Design review of the part built by this model. Coordinates are the model's own, in mm. A direction names the side the tool comes from. Coordinates: 2 decimals unless noted, no trailing zeros. Write each loop counter-clockwise with the first axis right and the second up, starting at its lowest first coordinate (ties: lowest second). Pieces come first, ordered by that corner, then holes. Notation, with made-up numbers: (19, 44.25) - (67, 44.25) arc R29 ccw to (67, 83.25) - close; hole circle Ø8 at (35, -9). An arc over 180 degrees is marked (long way). Answer as CSV lines item,"result". Start each with the question number.
Q1. Clearance check with flat-ended pins moving along their axes: pin 1 (2.5 mm diameter, centred on x = 0, y = 0, fed in from +Z); pin 2 (3 mm diameter, centred on x = 11.5, z = 4.5, fed in from -Y); pin 3 (1.5 mm diameter, centred on y = -3, z = 2, fed in from +X); pin 4 (3 mm diameter, centred on x = 6.5, z = 5, fed in from +Y). State where each tip first meets the part, or that it passes through.
Q2. We need section A-A (x = 0). Write out the cut boundary in (y, z), plus the area to 3 significant figures.
Q3. For line 1 along Y through (x, z) = (0, 3); line 2 along Y through (x, z) = (-9.5, 3.35); line 3 along X through (y, z) = (13.5, 0.7), list the stretches that pass through material, from the lowest coordinate up. Write a range as [from, to].
Q4. Mouldability with a two-part tool opening along X and no side actions: class faces 4 (the face through (0, 16.5, 3)), 5 (the face through (-5.089, 15.696, 2.712)), 6 (the face through (13.34, -9.71, 2.71)), 7 (the face through (-7.8, -12.8, 2.7)) as pulls with the +X half, pulls with the -X half, needs draft (parallel to the pull), parting line crosses it, or undercut.
Q5. Machinability: for faces 1 (the face through (1.2, -15, 2.7)), 2 (the face through (13.332, -2.12, 2.712)), 3 (the face through (-5.773, -13.85, 2.712)), which of the approach directions +Z, -Z, +X, -X, +Y, -Y give a long, thin tool a straight path to every point of the face, cutting with its end or side? Answer none if there is none.
Q6. We need section D-D (x = 9.5). Write out the cut boundary in (y, z).
Q7. We need section C-C (z = 2.25). State how many separate pieces and enclosed holes the cut face has, plus the area to 3 significant figures.
from build123d import *

# Parameters (mm, degrees)
SKETCH_1_R          = 13.5
EXTRUDE_1_DEPTH     = 5.5
EXTRUDE_START       = -5.5
EXTRUDE_2_DEPTH     = 5.5
SKETCH_7_R          = 2
CUT_EXTRUDE_1_DEPTH = 24.973944189
SKETCH_8_R          = 12.5
SKETCH_8_R_2        = 3
CUT_EXTRUDE_2_DEPTH = 4


with BuildPart() as part:
    # 草图1 → 凸台-拉伸1 (new body)
    with BuildSketch(Plane.XY):
        Circle(SKETCH_1_R)
    extrude(amount=EXTRUDE_1_DEPTH)

    # 草图6 → 凸台-拉伸2 (add)
    with BuildSketch(Plane.XY.offset(5.5).offset(EXTRUDE_START)):
        with BuildLine():
            Line((5.812072794, 15.460669773), (4.38548802, 15.924195265))
            ThreePointArc((4.38548802, 15.924195265), (3.48195608, 14.617198294), (2.719313259, 13.223287617))
            ThreePointArc((2.719313259, 13.223287617), (4.171729424, 12.83926297), (5.572482808, 12.296236634))
            ThreePointArc((5.572482808, 12.296236634), (5.774811944, 13.872204263), (5.812072794, 15.460669773))
        make_face()
        with BuildLine():
            Line((10.305219409, 12.907941468), (9.091693917, 13.789619346))
            ThreePointArc((9.091693917, 13.789619346), (7.828499702, 12.825798085), (6.67244119, 11.735779845))
            ThreePointArc((6.67244119, 11.735779845), (7.935100906, 10.921729424), (9.099492173, 9.972424088))
            ThreePointArc((9.099492173, 9.972424088), (9.778919397, 11.40873523), (10.305219409, 12.907941468))
        make_face()
        with BuildLine():
            Line((0.75, 16.5), (-0.75, 16.5))
            ThreePointArc((-0.75, 16.5), (-1.205425663, 14.97776529), (-1.5, 13.416407865))
            ThreePointArc((-1.5, 13.416407865), (0, 13.5), (1.5, 13.416407865))
            ThreePointArc((1.5, 13.416407865), (1.205425663, 14.97776529), (0.75, 16.5))
        make_face()
        with BuildLine():
            Line((13.789619346, 9.091693917), (12.907941468, 10.305219409))
            ThreePointArc((12.907941468, 10.305219409), (11.40873523, 9.778919397), (9.972424088, 9.099492173))
            ThreePointArc((9.972424088, 9.099492173), (10.921729424, 7.935100906), (11.735779845, 6.67244119))
            ThreePointArc((11.735779845, 6.67244119), (12.825798085, 7.828499702), (13.789619346, 9.091693917))
        make_face()
        with BuildLine():
            Line((15.924195265, 4.38548802), (15.460669773, 5.812072794))
            ThreePointArc((15.460669773, 5.812072794), (13.872204263, 5.774811944), (12.296236634, 5.572482808))
            ThreePointArc((12.296236634, 5.572482808), (12.83926297, 4.171729424), (13.223287617, 2.719313259))
            ThreePointArc((13.223287617, 2.719313259), (14.617198294, 3.48195608), (15.924195265, 4.38548802))
        make_face()
        with BuildLine():
            Line((16.5, -0.75), (16.5, 0.75))
            ThreePointArc((16.5, 0.75), (14.97776529, 1.205425663), (13.416407865, 1.5))
            ThreePointArc((13.416407865, 1.5), (13.5, 0), (13.416407865, -1.5))
            ThreePointArc((13.416407865, -1.5), (14.97776529, -1.205425663), (16.5, -0.75))
        make_face()
        with BuildLine():
            Line((15.460669773, -5.812072794), (15.924195265, -4.38548802))
            ThreePointArc((15.924195265, -4.38548802), (14.617198294, -3.48195608), (13.223287617, -2.719313259))
            ThreePointArc((13.223287617, -2.719313259), (12.83926297, -4.171729424), (12.296236634, -5.572482808))
            ThreePointArc((12.296236634, -5.572482808), (13.872204263, -5.774811944), (15.460669773, -5.812072794))
        make_face()
        with BuildLine():
            Line((12.907941468, -10.305219409), (13.789619346, -9.091693917))
            ThreePointArc((13.789619346, -9.091693917), (12.825798085, -7.828499702), (11.735779845, -6.67244119))
            ThreePointArc((11.735779845, -6.67244119), (10.921729424, -7.935100906), (9.972424088, -9.099492173))
            ThreePointArc((9.972424088, -9.099492173), (11.40873523, -9.778919397), (12.907941468, -10.305219409))
        make_face()
        with BuildLine():
            Line((9.091693917, -13.789619346), (10.305219409, -12.907941468))
            ThreePointArc((10.305219409, -12.907941468), (9.778919397, -11.40873523), (9.099492173, -9.972424088))
            ThreePointArc((9.099492173, -9.972424088), (7.935100906, -10.921729424), (6.67244119, -11.735779845))
            ThreePointArc((6.67244119, -11.735779845), (7.828499702, -12.825798085), (9.091693917, -13.789619346))
        make_face()
        with BuildLine():
            Line((4.38548802, -15.924195265), (5.812072794, -15.460669773))
            ThreePointArc((5.812072794, -15.460669773), (5.774811944, -13.872204263), (5.572482808, -12.296236634))
            ThreePointArc((5.572482808, -12.296236634), (4.171729424, -12.83926297), (2.719313259, -13.223287617))
            ThreePointArc((2.719313259, -13.223287617), (3.48195608, -14.617198294), (4.38548802, -15.924195265))
        make_face()
        with BuildLine():
            Line((-0.75, -16.5), (0.75, -16.5))
            ThreePointArc((0.75, -16.5), (1.205425663, -14.97776529), (1.5, -13.416407865))
            ThreePointArc((1.5, -13.416407865), (0, -13.5), (-1.5, -13.416407865))
            ThreePointArc((-1.5, -13.416407865), (-1.205425663, -14.97776529), (-0.75, -16.5))
        make_face()
        with BuildLine():
            Line((-5.812072794, -15.460669773), (-4.38548802, -15.924195265))
            ThreePointArc((-4.38548802, -15.924195265), (-3.48195608, -14.617198294), (-2.719313259, -13.223287617))
            ThreePointArc((-2.719313259, -13.223287617), (-4.171729424, -12.83926297), (-5.572482808, -12.296236634))
            ThreePointArc((-5.572482808, -12.296236634), (-5.774811944, -13.872204263), (-5.812072794, -15.460669773))
        make_face()
        with BuildLine():
            Line((-10.305219409, -12.907941468), (-9.091693917, -13.789619346))
            ThreePointArc((-9.091693917, -13.789619346), (-7.828499702, -12.825798085), (-6.67244119, -11.735779845))
            ThreePointArc((-6.67244119, -11.735779845), (-7.935100906, -10.921729424), (-9.099492173, -9.972424088))
            ThreePointArc((-9.099492173, -9.972424088), (-9.778919397, -11.40873523), (-10.305219409, -12.907941468))
        make_face()
        with BuildLine():
            Line((-13.789619346, -9.091693917), (-12.907941468, -10.305219409))
            ThreePointArc((-12.907941468, -10.305219409), (-11.40873523, -9.778919397), (-9.972424088, -9.099492173))
            ThreePointArc((-9.972424088, -9.099492173), (-10.921729424, -7.935100906), (-11.735779845, -6.67244119))
            ThreePointArc((-11.735779845, -6.67244119), (-12.825798085, -7.828499702), (-13.789619346, -9.091693917))
        make_face()
        with BuildLine():
            Line((-15.924195265, -4.38548802), (-15.460669773, -5.812072794))
            ThreePointArc((-15.460669773, -5.812072794), (-13.872204263, -5.774811944), (-12.296236634, -5.572482808))
            ThreePointArc((-12.296236634, -5.572482808), (-12.83926297, -4.171729424), (-13.223287617, -2.719313259))
            ThreePointArc((-13.223287617, -2.719313259), (-14.617198294, -3.48195608), (-15.924195265, -4.38548802))
        make_face()
        with BuildLine():
            Line((-16.5, 0.75), (-16.5, -0.75))
            ThreePointArc((-16.5, -0.75), (-14.97776529, -1.205425663), (-13.416407865, -1.5))
            ThreePointArc((-13.416407865, -1.5), (-13.5, 0), (-13.416407865, 1.5))
            ThreePointArc((-13.416407865, 1.5), (-14.97776529, 1.205425663), (-16.5, 0.75))
        make_face()
        with BuildLine():
            Line((-15.460669773, 5.812072794), (-15.924195265, 4.38548802))
            ThreePointArc((-15.924195265, 4.38548802), (-14.617198294, 3.48195608), (-13.223287617, 2.719313259))
            ThreePointArc((-13.223287617, 2.719313259), (-12.83926297, 4.171729424), (-12.296236634, 5.572482808))
            ThreePointArc((-12.296236634, 5.572482808), (-13.872204263, 5.774811944), (-15.460669773, 5.812072794))
        make_face()
        with BuildLine():
            Line((-12.907941468, 10.305219409), (-13.789619346, 9.091693917))
            ThreePointArc((-13.789619346, 9.091693917), (-12.825798085, 7.828499702), (-11.735779845, 6.67244119))
            ThreePointArc((-11.735779845, 6.67244119), (-10.921729424, 7.935100906), (-9.972424088, 9.099492173))
            ThreePointArc((-9.972424088, 9.099492173), (-11.40873523, 9.778919397), (-12.907941468, 10.305219409))
        make_face()
        with BuildLine():
            Line((-9.091693917, 13.789619346), (-10.305219409, 12.907941468))
            ThreePointArc((-10.305219409, 12.907941468), (-9.778919397, 11.40873523), (-9.099492173, 9.972424088))
            ThreePointArc((-9.099492173, 9.972424088), (-7.935100906, 10.921729424), (-6.67244119, 11.735779845))
            ThreePointArc((-6.67244119, 11.735779845), (-7.828499702, 12.825798085), (-9.091693917, 13.789619346))
        make_face()
        with BuildLine():
            Line((-4.38548802, 15.924195265), (-5.812072794, 15.460669773))
            ThreePointArc((-5.812072794, 15.460669773), (-5.774811944, 13.872204263), (-5.572482808, 12.296236634))
            ThreePointArc((-5.572482808, 12.296236634), (-4.171729424, 12.83926297), (-2.719313259, 13.223287617))
            ThreePointArc((-2.719313259, 13.223287617), (-3.48195608, 14.617198294), (-4.38548802, 15.924195265))
        make_face()
    extrude(amount=EXTRUDE_2_DEPTH)

    # 草图7 → 切除-拉伸1 (cut, through all)
    with BuildSketch(Plane(origin=(0, 0, 0), x_dir=(-1, 0, 0), z_dir=(0, 0, -1))):
        Circle(SKETCH_7_R)
    extrude(amount=-CUT_EXTRUDE_1_DEPTH, mode=Mode.SUBTRACT)

    # 草图8 → 切除-拉伸2 (cut)
    with BuildSketch(Plane(origin=(0, 0, 0), x_dir=(-1, 0, 0), z_dir=(0, 0, -1))):
        Circle(SKETCH_8_R)
        Circle(SKETCH_8_R_2, mode=Mode.SUBTRACT)
    extrude(amount=-CUT_EXTRUDE_2_DEPTH, mode=Mode.SUBTRACT)


solid = part.part
Results list:
1,pin 1,"passes through"
1,pin 2,"stops at y = -13.13"
1,pin 3,"stops at x = 15.04"
1,pin 4,"stops at y = 15.72"
2,outline,"(-16.5, 0) - (-12.5, 0) - (-12.5, 4) - (-3, 4) - (-3, 0) - (-2, 0) - (-2, 5.5) - (-16.5, 5.5) - close; (2, 0) - (3, 0) - (3, 4) - (12.5, 4) - (12.5, 0) - (16.5, 0) - (16.5, 5.5) - (2, 5.5) - close"
2,area,"83.5 mm2"
3,line 1,"y = [-16.5, -12.5], [-3, -2], [2, 3], [12.5, 16.5]"
3,line 2,"y = [-13.49, -10.77], [-9.59, -8.12], [8.12, 9.59], [10.77, 13.49]"
3,line 3,"x = [-9.49, -8.68], [-5.74, -2.86], [-1.49, 1.49], [2.86, 5.74], [8.68, 9.49]"
4,face 4,"needs draft"
4,face 5,"pulls with the -X half"
4,face 6,"pulls with the +X half"
4,face 7,"undercut"
5,face 1,"+Z, -Z, -Y"
5,face 2,"+Z, -Z, +X"
5,face 3,"+Z, -Z"
6,outline,"(-13.49, 0) - (-10.77, 0) - (-10.77, 5.5) - (-13.49, 5.5) - close; (-9.59, 0) - (-8.12, 0) - (-8.12, 4) - (8.12, 4) - (8.12, 0) - (9.59, 0) - (9.59, 5.5) - (-9.59, 5.5) - close; (10.77, 0) - (13.49, 0) - (13.49, 5.5) - (10.77, 5.5) - close"
7,separate pieces,"2"
7,enclosed holes,"2"
7,area,"240 mm2"
